Part print with two shaded views. Sizes in mm from the minimum x, y, z corner. Round coordinates to 2 decimals unless told otherwise and drop trailing zeros. Loops run counter-clockwise (first coordinate to the right, second up) from the corner with the lowest first, then second, coordinate; pieces in that order, holes last. Notation, with made-up numbers: (60.5, 71) -> (104.5, 71) arc R20 cw to (104.5, 107) -> close; hole circle Ø4 at (48.5, -19.5). An arc over 180 degrees is marked (long way). Use a Markdown table: item, result. Add a question column.
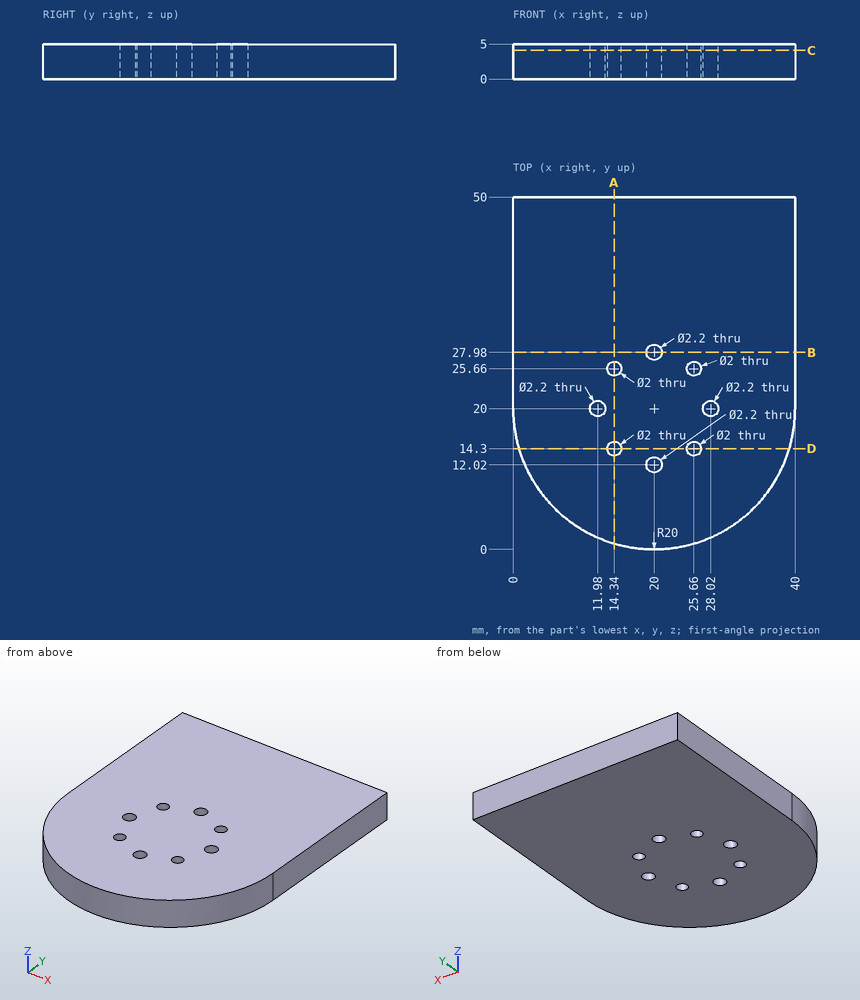
1) Cut at C-C on z = 4.1. Count the separate pieces of the cut face and the enclosed holes in it, and give its area (3 significant figures).
2) Cut at B-B on y = 27.98. Write the cut outline in (x, z), and give its area (3 significant figures).
3) Pin check, flat tips, straight feed: pin 1 Ø5 at (x, y) = (7.5, 28.5) entering from -Z; pin 2 Ø2 at (x, y) = (20, 27.98) entering from +Z. Stop position of each tip, or through.
4) Cut at D-D on y = 14.3. Write the cut outline in (x, z), and give its area (3 significant figures).
5) Wall check: probe 1 along X at (y, z) = (20, 2.2); probe 2 along X at (y, z) = (25.66, 3.65); probe 3 along Y at (x, z) = (25.66, 1.4). Give the ranges that are in metal, low to high. Write a range as from..to.
6) Cut at A-A on x = 14.34. Write the cut outline in (y, z), and give its area (3 significant figures).
Established:
| question | item | result |
|---|---|---|
| 1 | separate pieces | 1 |
| 1 | enclosed holes | 8 |
| 1 | area | 1,800 mm^2 |
| 2 | outline | (0, 0) -> (18.9, 0) -> (18.9, 5) -> (0, 5) -> close; (21.1, 0) -> (40, 0) -> (40, 5) -> (21.1, 5) -> close |
| 2 | area | 189 mm^2 |
| 3 | pin 1 | stops at z = 0 |
| 3 | pin 2 | passes through |
| 4 | outline | (0.83, 0) -> (13.34, 0) -> (13.34, 5) -> (0.83, 5) -> close; (15.34, 0) -> (24.66, 0) -> (24.66, 5) -> (15.34, 5) -> close; (26.66, 0) -> (39.17, 0) -> (39.17, 5) -> (26.66, 5) -> close |
| 4 | area | 172 mm^2 |
| 5 | probe 1 | x = 0..10.88, 13.08..26.92, 29.12..40 |
| 5 | probe 2 | x = 0..13.34, 15.34..24.66, 26.66..40 |
| 5 | probe 3 | y = 0.82..13.3, 15.3..24.66, 26.66..50 |
| 6 | outline | (0.82, 0) -> (13.3, 0) -> (13.3, 5) -> (0.82, 5) -> close; (15.3, 0) -> (24.66, 0) -> (24.66, 5) -> (15.3, 5) -> close; (26.66, 0) -> (50, 0) -> (50, 5) -> (26.66, 5) -> close |
| 6 | area | 226 mm^2 |
